Read the model definition and answer for the solid it produces. Units are mm, in the model's axes. Coordinates: 2 decimals unless noted, no trailing zeros. Write each loop counter-clockwise with the first axis right and the second up, starting at its lowest first coordinate (ties: lowest second). Pieces come first, ordered by that corner, then holes. Notation, with made-up numbers: M 89.25,15 L 148.25,15 A16 ccw 148.25,39 Z; hole C 19,2 d6. An arc over 180 degrees is marked long. Write item = value, one per line.
from build123d import *

# Parameters (mm, degrees)
ESQUISSE1_W             = 90
ESQUISSE1_H             = 2
EXTRU_MINCE1_DEPTH      = 25
CONG_1_R                = 2
CONG_2_R                = 2
CONG_3_R                = 2
CONG_4_R                = 2
ESQUISSE2_R             = 2.25
ENL_V_MAT_EXTRU_1_DEPTH = 10


with BuildPart() as part:
    # Esquisse1 → Extru.-Mince1 (new body)
    with BuildSketch(Plane.XY):
        with Locations((45, -1)):
            Rectangle(ESQUISSE1_W, ESQUISSE1_H)
    extrude(amount=EXTRU_MINCE1_DEPTH)

    # Congé1
    cong_1_edges = [part.edges().sort_by_distance(p)[0] for p in [
        (90, -1, 25),
    ]]
    fillet(cong_1_edges, radius=CONG_1_R)

    # Congé2
    cong_2_edges = [part.edges().sort_by_distance(p)[0] for p in [
        (90, -1, 0),
    ]]
    fillet(cong_2_edges, radius=CONG_2_R)

    # Congé3
    cong_3_edges = [part.edges().sort_by_distance(p)[0] for p in [
        (0, -1, 0),
    ]]
    fillet(cong_3_edges, radius=CONG_3_R)

    # Congé4
    cong_4_edges = [part.edges().sort_by_distance(p)[0] for p in [
        (0, -1, 25),
    ]]
    fillet(cong_4_edges, radius=CONG_4_R)

    # Esquisse2 → Enlèv. mat.-Extru.1 (cut)
    with BuildSketch(Plane(origin=(0, 0, 0), x_dir=(1, 0, 0), z_dir=(0, 1, 0))):
        with Locations(Location((82, -12.5, 0), (0, 0, 270))):
            Circle(ESQUISSE2_R)
        with Locations(Location((8, -12.5, 0), (0, 0, 270))):
            Circle(ESQUISSE2_R)
    extrude(amount=-ENL_V_MAT_EXTRU_1_DEPTH, mode=Mode.SUBTRACT)


solid = part.part
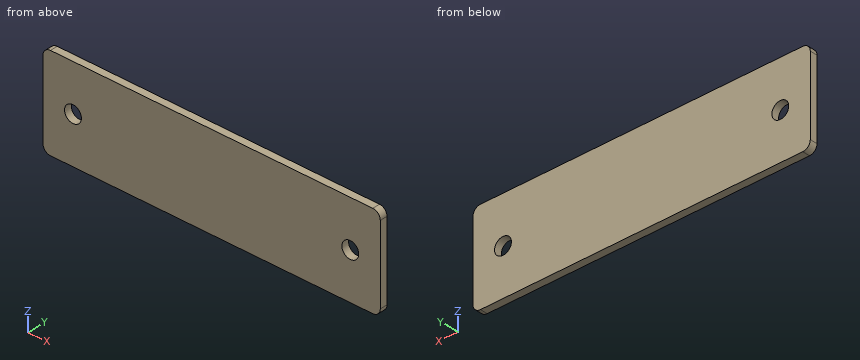
Item 1: A flat-ended cylindrical pin translates along its axis: pin 1 (1 mm diameter, centred on x = 77, z = 9.5, fed in from +Y). Find the tip coordinate at first contact, or state that the pin passes through.
Worked answers:
pin_1 = 0
Item 2: Find section D-D (x = 9.5). Determine the outline of the cut face in (y, z).
Worked answers:
outline = M -2,0 L 0,0 L 0,10.82 L -2,10.82 Z; M -2,14.18 L 0,14.18 L 0,25 L -2,25 Z
Item 3: Find section B-B (x = 82). Determine the outline of the cut face in (y, z).
Worked answers:
outline = M -2,0 L 0,0 L 0,10.25 L -2,10.25 Z; M -2,14.75 L 0,14.75 L 0,25 L -2,25 Z
Item 4: Consider line 1 along X through (y, z) = (-1.5, 12.5); line 2 along Z through (x, y) = (84, -0.35). Determine where each line is inside the solid, lowest interval first. Write a range as from..to.
Worked answers:
line_1 = 0..5.75, 10.25..79.75, 84.25..90
line_2 = 0..11.47, 13.53..25
Item 5: Find section A-A (y = -0.7). Determine the outline of the cut face in (x, z).
Worked answers:
outline = M 0,2 A2 ccw 2,0 L 88,0 A2 ccw 90,2 L 90,23 A2 ccw 88,25 L 2,25 A2 ccw 0,23 Z; hole C 8,12.5 d4.5; hole C 82,12.5 d4.5
Item 6: Find section C-C (z = 12.5). Determine the outline of the cut face in (x, y), and give its area (3 significant figures).
Worked answers:
outline = M 0,-2 L 5.75,-2 L 5.75,0 L 0,0 Z; M 10.25,-2 L 79.75,-2 L 79.75,0 L 10.25,0 Z; M 84.25,-2 L 90,-2 L 90,0 L 84.25,0 Z
area = 162 mm²
